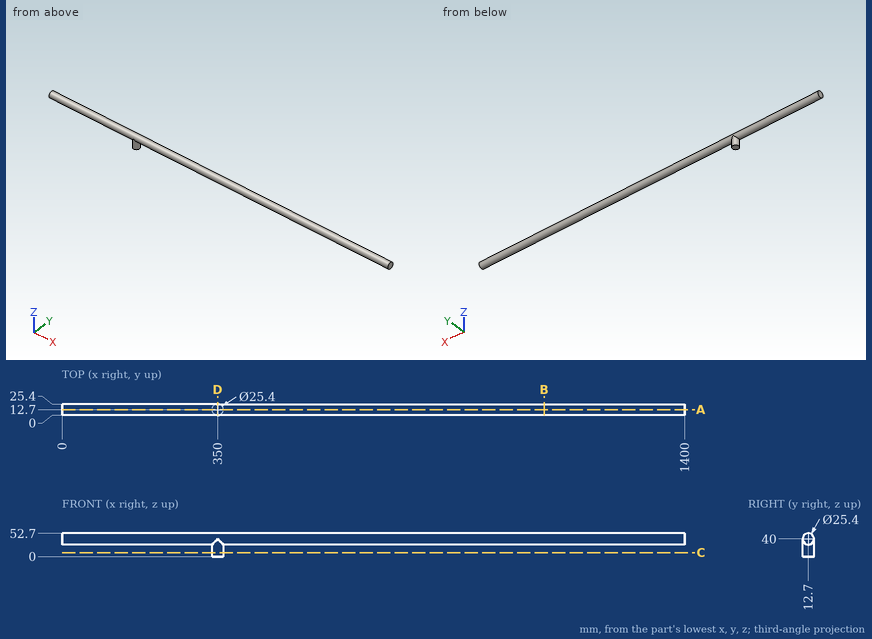
Input: dimensioned drawing with shaded views. Units: mm. Origin: part minimum x, y, z. Give positions to 0.01 mm unless a question says otherwise; leave off trailing zeros. Write each loop counter-clockwise with the first axis right and the second up, starting at its lowest first coordinate (ties: lowest second). Pieces come first, ordered by that corner, then holes.
1. Section query C-C (z = 9). Return the cut outline in (x, y), then the cut area to 3 significant figures.
2. Material intervals for line 1 along X through (y, z) = (12.75, 13.5); line 2 along X through (y, z) = (15, 20); line 3 along Z through (x, y) = (748, 15.25), sorted ascending.
3. Section query D-D (x = 350). Return the cut outline in (y, z).
4. Section query B-B (x = 1084). Return the cut outline in (y, z), then the cut area to 3 significant figures.
5. Section query A-A (y = 12.7). Return the cut outline in (x, z).
6. First-contact query: pin 1 (8 mm diameter, centred on x = 682, y = 15.5, fed in from -Z); pin 2 (1.5 mm diameter, centred on x = 704.5, y = 21, fed in from +Z); pin 3 (1 mm diameter, centred on y = 8.5, z = 15.5, fed in from -X). Flat tips, straight axial feed; report the tip coordinate or a pass-through.
Output values:
1. outline: circle Ø25.4 at (350, 12.7)
1. area: 507 mm2
2. line 1: x = 337.3 to 362.7
2. line 2: x = 337.51 to 362.49
2. line 3: z = 27.56 to 52.44
3. outline: (0, 0) - (25.4, 0) - (25.4, 40) arc R12.7 ccw to (0, 40) - close
4. outline: circle Ø25.4 at (12.7, 40)
4. area: 507 mm2
5. outline: (0, 27.3) - (337.3, 27.3) - (337.3, 0) - (362.7, 0) - (362.7, 27.3) - (1400, 27.3) - (1400, 52.7) - (0, 52.7) - close
6. pin 1: stops at z = 27.3
6. pin 2: stops at z = 50.21
6. pin 3: stops at x = 337.85
